Verification items for this drawing (mm, ordinates from the low corner). Give positions to 0.01 mm unless a question says otherwise; leave off trailing zeros. Order: outer loops, then holes, each group sorted by start corner. A loop starts at its lowest first (then second) coordinate and runs counter-clockwise, first axis right, second up.
(1) Sectioned sample at D-D on x = 17.75. Record the cut outline in (y, z) (3 decimals).
(2) Sectioned sample at A-A on y = 50. Record the cut outline in (x, z).
(3) Sectioned sample at B-B on z = 64.5. Record the cut outline in (x, y), plus the area to 3 significant figures.
(4) Mould release check, pull along Y, two halves, no side actions. Record for the marked faces 1, 2 and 3: pulls with the +Y half, pulls with the -Y half, needs draft (parallel to the pull), parting line crosses it, or undercut.
(5) Sectioned sample at C-C on x = 3.25. Record the cut outline in (y, z) (3 decimals).
(6) Scan lines: L1, parallel to X at y = 6, z = 52; L2, parallel to Y at x = 2.75, z = 64.5; L3, parallel to Z at x = 6.75, y = 44. Record each from-to range of solid material in increasing order.
(7) Gauge pin test, flat ends, axial feed: pin 1 (6 mm diameter, centred on x = 6, z = 59, fed in from -Y); pin 2 (7.5 mm diameter, centred on y = 52, z = 48, fed in from -X); pin 3 (8 mm diameter, centred on x = 14, z = 87, fed in from -Y). Record the tip position at first contact, or that the pin passes through.
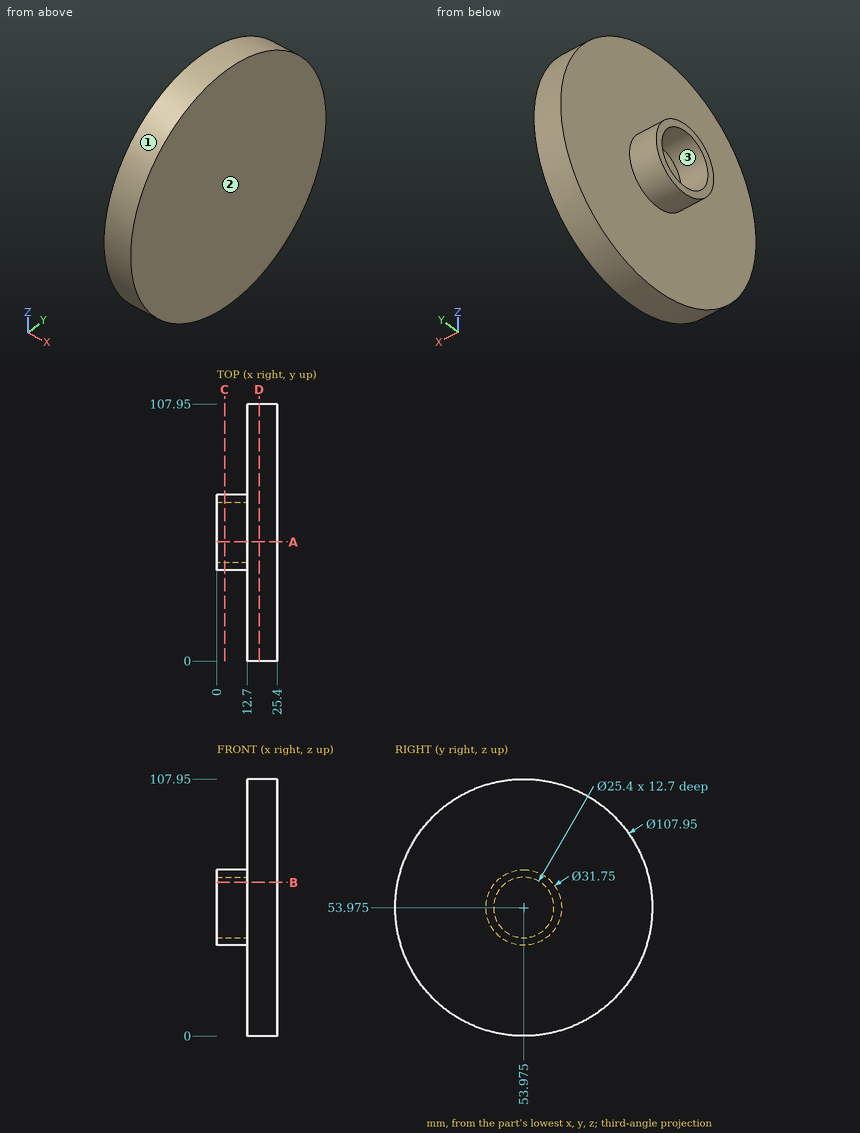
Ans:
1. outline: circle Ø107.95 at (53.975, 53.975)
2. outline: (0, 38.61) - (12.7, 38.61) - (12.7, 0.15) - (25.4, 0.15) - (25.4, 107.8) - (12.7, 107.8) - (12.7, 69.34) - (0, 69.34) - (0, 66.04) - (12.7, 66.04) - (12.7, 41.91) - (0, 41.91) - close
3. outline: (0, 42.09) - (12.7, 42.09) - (12.7, 1.04) - (25.4, 1.04) - (25.4, 106.91) - (12.7, 106.91) - (12.7, 65.86) - (0, 65.86) - (0, 61.08) - (12.7, 61.08) - (12.7, 46.87) - (0, 46.87) - close
3. area: 1,470 mm2
4. face 1: parting line crosses it
4. face 2: needs draft
4. face 3: undercut
5. outline: circle Ø31.75 at (53.975, 53.975); hole circle Ø25.4 at (53.975, 53.975)
6. L1: x = 12.7 to 25.4
6. L2: y = 42.09 to 46.87, 61.08 to 65.86
6. L3: z = 41.63 to 46.11, 61.84 to 66.32
7. pin 1: stops at y = 38.23
7. pin 2: stops at x = 12.7
7. pin 3: stops at y = 8.47
